Work out the finished part from the listing and answer in its coordinate system (mm). Coordinates: 2 decimals unless noted, no trailing zeros. Write each loop counter-clockwise with the first axis right and the second up, starting at its lowest first coordinate (ties: lowest second). Pieces come first, ordered by that corner, then holes. Notation, with made-up numbers: (7, -28.5) - (37, -28.5) arc R15 ccw to (37, -16.5) - close; hole circle Ø5 at (74.25, -6). An arc over 180 degrees is marked (long way). One line per item, written item: value.
```python
from build123d import *

# Parameters (mm, degrees)
EXTRUDE_1_DEPTH        = 9
M12X1_25_1_D           = 10.8
M12X1_25_1_DEPTH       = 27.75
M12X1_25_1_CBORE_D     = 12
M12X1_25_1_CBORE_DEPTH = 24
M12X1_25_1_TIP         = 3.244647343


with BuildPart() as part:
    # 草图1 → 拉伸1 (new body)
    with BuildSketch(Plane.XY):
        Polygon((-5.484827557, 9.5), (5.484827557, 9.5), (10.969655115, 0), (5.484827557, -9.5), (-5.484827557, -9.5), (-10.969655115, 0), align=None)
    extrude(amount=EXTRUDE_1_DEPTH)

    # M12x1.25 螺纹孔1
    with Locations(Plane(origin=(0.002521047, 0, 9), x_dir=(1, 0, 0), z_dir=(0, 0, 1))):
        with Locations((0, 0)):
            CounterBoreHole(M12X1_25_1_D / 2, M12X1_25_1_CBORE_D / 2, M12X1_25_1_CBORE_DEPTH, depth=M12X1_25_1_DEPTH)
            with Locations((0, 0, -(M12X1_25_1_DEPTH + M12X1_25_1_TIP / 2))):  # 118° drill point
                Cone(0, M12X1_25_1_D / 2, M12X1_25_1_TIP, mode=Mode.SUBTRACT)


solid = part.part
```
Item 1: Section D-D, the plane y = -6.25 is taken. Determine the outline of the cut face in (x, z).
Evaluation:
outline: (-7.36, 0) - (7.36, 0) - (7.36, 9) - (-7.36, 9) - close
Item 2: Section A-A, the plane x = 0.5 is taken. Determine the outline of the cut face in (y, z), then the cut area to 3 significant figures.
Evaluation:
outline: (-9.5, 0) - (-5.98, 0) - (-5.98, 9) - (-9.5, 9) - close; (5.98, 0) - (9.5, 0) - (9.5, 9) - (5.98, 9) - close
area: 63.4 mm2
Item 3: Consider probe 1 along Y at (x, z) = (1.5, 4.5); probe 2 along Y at (x, z) = (-4.5, 1); probe 3 along X at (y, z) = (4.5, 7.5). Determine where each line is inside the solid, lowest interval first.
Evaluation:
probe 1: y = -9.5 to -5.81, 5.81 to 9.5
probe 2: y = -9.5 to -3.97, 3.97 to 9.5
probe 3: x = -8.37 to -3.97, 3.97 to 8.37
Item 4: Section C-C, the plane y = 4.5 is taken. Determine the outline of the cut face in (x, z), then the cut area to 3 significant figures.
Evaluation:
outline: (-8.37, 0) - (-3.97, 0) - (-3.97, 9) - (-8.37, 9) - close; (3.97, 0) - (8.37, 0) - (8.37, 9) - (3.97, 9) - close
area: 79.3 mm2
Item 5: Section B-B, the plane z = 5 is taken. Determine the outline of the cut face in (x, y).
Evaluation:
outline: (-10.97, 0) - (-5.48, -9.5) - (5.48, -9.5) - (10.97, 0) - (5.48, 9.5) - (-5.48, 9.5) - close; hole circle Ø12 at (0, 0)
Item 6: Determine the mould class of faces 1 (the face through (-5, 4, 0)), 2 (the face through (8.2, 4.8, 4.4)), 3 (the face through (-4.76, -3.65, 4.56)) for opening direction X: +X half, -X half, draft (parallel to the pull), parting line (faces both ways), or undercut.
Evaluation:
face 1: draft
face 2: +X half
face 3: undercut
